```python
from build123d import *

# Parameters (mm, degrees)
PAD004_DEPTH            = 102
SKETCH006_R             = 2.75
POCKET001_DEPTH         = 19.817629
SKETCH007_R             = 5
POCKET002_DEPTH         = 14.817629
BODY002_PLACEMENT_ANGLE = 180


with BuildPart() as part:
    # Sketch004 → Pad004 (new body)
    with BuildSketch(Plane.YZ):
        Polygon((-6.970253, 4), (-6.970253, 21.219848), (-11.970253, 21.219848), (-20, 4), (-20, 0), (0, 0), (0, 4), align=None)
    extrude(amount=-PAD004_DEPTH)

    # Sketch006 (on Face3 of Pad004) → Pocket001 (cut, through all)
    with BuildSketch(Plane(origin=(0, -17.959965, 8.374869), x_dir=(0, -0.422618, -0.906308), z_dir=(0, -0.906308, 0.422618))):
        with Locations((-5.172866, -33.45)):
            Circle(SKETCH006_R)
        with Locations((-5.172866, -71.55)):
            Circle(SKETCH006_R)
    extrude(amount=-POCKET001_DEPTH, mode=Mode.SUBTRACT)

    # Sketch007 (on Face9 of Pocket001) → Pocket002 (cut, through all)
    with BuildSketch(Plane(origin=(0, -13.428426, 6.261778), x_dir=(0, -0.422618, -0.906308), z_dir=(0, -0.906308, 0.422618))):
        with Locations((-5.172866, -33.45)):
            Circle(SKETCH007_R)
        with Locations((-5.172866, -71.55)):
            Circle(SKETCH007_R)
    extrude(amount=-POCKET002_DEPTH, mode=Mode.SUBTRACT)


with BuildPart() as part_1:
    # Body002 placement: moved
    add(part.part.moved(Location((2, 35, 36))).rotate(Axis((2, 35, 36), (0, 0, 1)), BODY002_PLACEMENT_ANGLE))


solid = part_1.part
```
Input: part model. Units: mm. Frame: model coordinates. A direction names the side the tool comes from. Round coordinates to 2 decimals unless told otherwise and drop trailing zeros. Loops run counter-clockwise (first coordinate to the right, second up) from the corner with the lowest first, then second, coordinate; pieces in that order, holes last. Notation, with made-up numbers: (-2, -2.75) -> (41, -2.75) arc R17 cw to (41, 1.25) -> close; hole circle Ø10 at (53, 74). An arc over 180 degrees is marked (long way). Use one line per item in the form item = value. Start each with the question number.
Item 1: Material intervals for L1, parallel to Y at x = 75, z = 51; L2, parallel to Z at x = 13, y = 41.5; L3, parallel to Z at x = 33, y = 48, sorted ascending. Write a range as from..to.
Item 2: Contact query for flat-ended pins moving along their axis: pin 1 Ø2 at (x, z) = (13, 51.5) entering from +Y; pin 2 Ø5.5 at (x, y) = (93, 37) entering from +Z; pin 3 Ø12 at (x, z) = (82, 49) entering from -Y. Output: stop coordinate, or through.
Item 3: Section query A-A on x = 14. Return the cut outline in (y, z), then the cut area to 3 significant figures.
Item 4: Set-up query: faces 1 (the face through (52, 55, 38)), 2 (the face through (75.7, 47.15, 45)), 3 (the face through (17, 38, 40)). Return all of +Z, -Z, +X, -X, +Y, -Y with unobstructed straight access to the full face (end or side cutting, diameter ignored); none if empty.
Item 5: Section query D-D on z = 54.75. Return the cut outline in (x, y), then the cut area to 3 significant figures.
Item 6: Section query C-C on y = 53.5. Return the cut outline in (x, z), then the cut area to 3 significant figures.
Item 7: Mould query, pull axis Y, two halves, no side actions, for faces 4 (the face through (52, 35, 38)), 5 (the face through (37.6, 47.15, 45)), 6 (the face through (37.365, 43.094, 40.386)), 7 (the face through (90, 38, 40)). Classes: pulls with the +Y half, pulls with the -Y half, needs draft (parallel to the pull), parting line crosses it, or undercut.
Item 8: Section query B-B on z = 47.5. Count the separate pieces of the cut face and the enclosed holes in it, then the cut area to 3 significant figures.
Ans:
q1.L1 = 41.97..43.6, 44.35..49.4
q1.L2 = 36..40
q1.L3 = 36..42.96, 43.18..46.39, 49.15..55.01
q2.pin_1 = 50.1
q2.pin_2 = 40
q2.pin_3 = 41.97
q3.outline = (35, 36) -> (55, 36) -> (55, 40) -> (46.97, 57.22) -> (41.97, 57.22) -> (41.97, 40) -> (35, 40) -> close
q3.area = 235 mm^2
q4.face_1 = +Z, -Z, +X, -X, +Y
q4.face_2 = none
q4.face_3 = +Z, +X, -X, -Y
q5.outline = (2, 41.97) -> (104, 41.97) -> (104, 48.12) -> (2, 48.12) -> close
q5.area = 627 mm^2
q6.outline = (2, 36) -> (104, 36) -> (104, 43.22) -> (2, 43.22) -> close
q6.area = 736 mm^2
q7.face_4 = pulls with the -Y half
q7.face_5 = undercut
q7.face_6 = undercut
q7.face_7 = needs draft
q8.separate_pieces = 3
q8.enclosed_holes = 0
q8.area = 839 mm^2
